Input: part model. Units: mm. Frame: model coordinates. A direction names the side the tool comes from. Give positions to 0.01 mm unless a question says otherwise; leave off trailing zeros. Write each loop counter-clockwise with the first axis right and the second up, starting at its lowest first coordinate (ties: lowest second). Pieces come first, ordered by that corner, then holes. Notation, with made-up numbers: (-36.5, -8.5) -> (-10.5, -8.5) arc R19 ccw to (-10.5, 20.5) -> close; hole circle Ø4 at (5.5, 15). An arc over 180 degrees is marked (long way). Return JSON: item names as keys, results as strings. Group by question number.
Item 1: Set-up query: faces 1 (the face through (-16, -15, 0)), 2 (the face through (17.55, -10.2, -10.64)), 3 (the face through (6.04, 19.38, -10.64)). Return all of +Z, -Z, +X, -X, +Y, -Y with unobstructed straight access to the full face (end or side cutting, diameter ignored); none if empty.
Item 2: Pin query (flat end, axial travel): P1, Ø5, axis at x = -11.5, y = 26, coming from the -Z side; P2, Ø5, axis at x = 9.5, z = 57.5, coming from the -Y side; P3, Ø8, axis at y = -14.5, z = 131, coming from the +X side. Return the tip coordinate at first contact, or that it passes through.
Item 3: Section A-A, the plane z = 47.5. Return loops of the section in (x, y).
Item 4: Section C-C, the plane x = -28.5. Return loops of the section in (y, z), then the cut area to 3 significant figures.
Item 5: Line query: line 1 (Z direction, x = 15.5, y = 18); line 2 (X direction, y = -10, z = 36.5); line 3 (Y direction, x = 9.5, z = 133). Output: solid intervals per line, ascending. Write a range as [from, to].
Item 6: Section B-B, the plane y = -13.5. Return loops of the section in (x, z).
from build123d import *

# Parameters (mm, degrees)
F1_DEPTH = 152.4
F3_DEPTH = 173.99


with BuildPart() as f1:
    # F0 (on Top) → F1 (new body)
    with BuildSketch(Plane.XY):
        Polygon((24.0552005179, -24.0552005179), (34.0191908181, 0), (24.0552005179, 24.0552005179), (0, 34.0191908181), (-24.0552005179, 24.0552005179), (-34.0191908181, 0), (-24.0552005179, -24.0552005179), (0, -34.0191908181), align=None)
    extrude(amount=F1_DEPTH)

    # F2 (on face) → F3 (join)
    with BuildSketch(Plane.XY.offset(152.4)):
        Polygon((-3.4393439428, 22.2672511014), (-19.5536338125, 11.1944166036), (-20.9436385999, -8.3080419212), (-6.5626563492, -21.5543754261), (12.7601399862, -18.5698246061), (22.4742906526, -1.6018171023), (15.2648420656, 16.5723913507), align=None)
    extrude(amount=-F3_DEPTH)


solid = f1.part
Answer below:
{
 "1": {"face 1": "-Z", "face 2": "-Z, +X, -Y", "face 3": "-Z, +X, +Y"},
 "2": {"P1": "stops at z = 0", "P2": "stops at y = -31.12", "P3": "stops at x = 29.67"},
 "3": {"outline": "(-34.02, 0) -> (-24.06, -24.06) -> (0, -34.02) -> (24.06, -24.06) -> (34.02, 0) -> (24.06, 24.06) -> (0, 34.02) -> (-24.06, 24.06) -> close"},
 "4": {"outline": "(-13.32, 0) -> (13.32, 0) -> (13.32, 152.4) -> (-13.32, 152.4) -> close", "area": "4,060 mm2"},
 "5": {"line 1": "z = [0, 152.4]", "line 2": "x = [-29.88, 29.88]", "line 3": "y = [-30.08, 30.08]"},
 "6": {"outline": "(-28.43, 0) -> (-15.31, 0) -> (-15.31, -21.59) -> (15.66, -21.59) -> (15.66, 0) -> (28.43, 0) -> (28.43, 152.4) -> (-28.43, 152.4) -> close"}
}
